Here's how the part is built. I have some questions about the finished solid (model axes, mm). Face numbers are marked on the shaded views. A direction names the side the tool comes from. Round coordinates to 2 decimals unless told otherwise and drop trailing zeros. Order: outer loops, then holes, each group sorted by start corner. A loop starts at its lowest first (then second) coordinate and runs counter-clockwise, first axis right, second up.
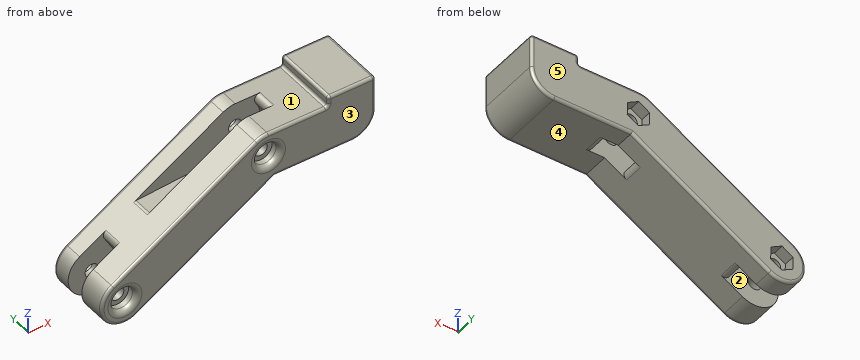
```python
from build123d import *

# Parameters (mm, degrees)
SKETCH1_R               = 1.2
BOSS_EXTRUDE1_DEPTH     = 12
CUT_EXTRUDE1_DEPTH      = 2.5
CUT_EXTRUDE1_DEPTH_BACK = 1
CUT_EXTRUDE2_DEPTH      = 2
SKETCH5_R               = 2.05
CUT_EXTRUDE3_DEPTH      = 2
FILLET1_R               = 1
FILLET2_R               = 0.5


with BuildPart() as part:
    # Sketch1 → Boss-Extrude1 (new body)
    with BuildSketch(Plane(origin=(0, 0, 0), x_dir=(1, 0, 0), z_dir=(0, 1, 0))):
        with BuildLine():
            Line((1.323018794, 17.222814504), (26.105840038, 2.488576956))
            Line((26.105840038, 2.488576956), (39.937870576, 2.488576956))
            ThreePointArc((39.937870576, 2.488576956), (42.943074396, 1.243780776), (44.187870576, -1.761423044))
            Line((44.187870576, -1.761423044), (44.187870576, -7.85))
            Line((44.187870576, -7.85), (35.687870576, -7.85))
            Line((35.687870576, -7.85), (35.687870576, -6.011423044))
            Line((35.687870576, -6.011423044), (24.937870576, -6.011423044))
            ThreePointArc((24.937870576, -6.011423044), (23.811655258, -5.859488326), (22.76596286, -5.414547306))
            Line((22.76596286, -5.414547306), (-3.020796638, 9.91656598))
            ThreePointArc((-3.020796638, 9.91656598), (-4.502013184, 15.741597958), (1.323018794, 17.222814504))
        make_face()
        with Locations(Location((-0.848888922, 13.569690242, 0), (0, 0, 270))):
            Circle(SKETCH1_R, mode=Mode.SUBTRACT)
        with Locations(Location((24.937870576, -1.761423044, 0), (0, 0, 270))):
            Circle(SKETCH1_R, mode=Mode.SUBTRACT)
    extrude(amount=BOSS_EXTRUDE1_DEPTH)

    # Sketch3 → Cut-Extrude1 (cut, two sides: drawn at the far end of the back side and taken through both)
    with BuildSketch(Plane(origin=(0, 6, 0), x_dir=(1, 0, 0), z_dir=(0, 1, 0)).offset(-CUT_EXTRUDE1_DEPTH_BACK)):
        with BuildLine():
            Line((-22.892544244, 0.947199994), (-3.741433166, 17.016890236))
            ThreePointArc((-3.741433166, 17.016890236), (2.065644543, 16.998318931), (3.019125003, 11.270023249))
            Line((3.019125003, 11.270023249), (-1.084785494, 4.367292117))
            ThreePointArc((-1.084785494, 4.367292117), (-0.38864398, 4.483185905), (0.317056148, 4.488816704))
            Line((0.317056148, 4.488816704), (25.254926724, 2.72739366))
            ThreePointArc((25.254926724, 2.72739366), (28.925298394, 0.324342858), (28.805884501, -4.061090037))
            Line((28.805884501, -4.061090037), (16.029956762, -25.550056285))
            ThreePointArc((16.029956762, -25.550056285), (9.862275844, -27.118403217), (8.293928913, -20.950722299))
            Line((8.293928913, -20.950722299), (17.339631919, -5.735951945))
            Line((17.339631919, -5.735951945), (-0.317056148, -4.488816704))
            ThreePointArc((-0.317056148, -4.488816704), (-2.876129239, -3.460907482), (-4.354991754, -1.1331579))
            Line((-4.354991754, -1.1331579), (-9.756802736, -10.218942999))
            ThreePointArc((-9.756802736, -10.218942999), (-15.508332614, -12.006129032), (-17.885892009, -6.472473713))
            ThreePointArc((-17.885892009, -6.472473713), (-23.730198417, -5.017065706), (-22.892544244, 0.947199994))
        make_face()
    extrude(amount=CUT_EXTRUDE1_DEPTH + CUT_EXTRUDE1_DEPTH_BACK, mode=Mode.SUBTRACT)

    # Sketch4 → Cut-Extrude2 (cut)
    with BuildSketch(Plane(origin=(0, 12, 0), x_dir=(1, 0, 0), z_dir=(0, 1, 0))):
        Polygon((22.952804904, -0.581233393), (22.923263521, -2.890445518), (24.908329193, -4.07063517), (26.922936248, -2.941612695), (26.952477631, -0.63240057), (24.967411959, 0.547789081), align=None)
        Polygon((1.13617675, 12.389500591), (1.165718133, 14.698712717), (-0.819347539, 15.878902368), (-2.833954594, 14.749879893), (-2.863495977, 12.440667768), (-0.878430305, 11.260478117), align=None)
    extrude(amount=-CUT_EXTRUDE2_DEPTH, mode=Mode.SUBTRACT)

    # Sketch5 → Cut-Extrude3 (cut)
    with BuildSketch(Plane.XZ):
        with Locations(Location((-0.848888922, -13.569690242, 0), (0, 0, 270))):
            Circle(SKETCH5_R)
        with Locations(Location((24.937870576, 1.761423044, 0), (0, 0, 270))):
            Circle(SKETCH5_R)
    extrude(amount=-CUT_EXTRUDE3_DEPTH, mode=Mode.SUBTRACT)

    # Fillet1
    # the kernel refuses this fillet: 1 mm, written as the material it takes off along each edge
    with BuildSketch(Plane(origin=(26.416890522, 8.5, -2.488576956), x_dir=(1, 0, 0), z_dir=(0, -1, 0)), Plane(origin=(2.594323181, 8.5, -16.466980426), x_dir=(0.8595586499303869, 0, 0.511037109542791), z_dir=(0, -1, 0))) as fillet1_piece_1:
        with BuildLine():
            CenterArc((2.958039892, 1), FILLET1_R, 143.77845338, 126.22154662)
            ThreePointArc((2.151301739, 1.590909091), (1.196627809, 0.631863865), (0, 0))
            Line((0, 0), (2.958039892, 0))
        make_face()
    extrude(amount=3.5, mode=Mode.SUBTRACT)
    with BuildSketch(Plane(origin=(27.64634461, 5, 6.011423044), x_dir=(1, 0, 0), z_dir=(0, 1, 0))) as fillet1_piece_2:
        with BuildLine():
            CenterArc((FILLET1_R * 1.75792205647, FILLET1_R), FILLET1_R, 149.267064192, 120.732935808)
            Line((FILLET1_R * 0.89836340654, FILLET1_R * 1.51103710954), (0, 0))
            Line((0, 0), (FILLET1_R * 1.75792205647, 0))
        make_face()
    extrude(amount=3.5, mode=Mode.SUBTRACT)
    with BuildSketch(Plane(origin=(6.889434617, 8.5, -4.024593471), x_dir=(-0.8595586499303914, 0, -0.5110371095427833), z_dir=(0, -1, 0))) as fillet1_piece_3:
        with BuildLine():
            CenterArc((FILLET1_R * 0.237244349344, FILLET1_R), FILLET1_R, 243.307295898, 26.692704102)
            Line((-FILLET1_R * 0.211960885996, FILLET1_R * 0.10657140378), (0, 0))
            Line((0, 0), (FILLET1_R * 0.237244349344, 0))
        make_face()
    extrude(amount=3.5, mode=Mode.SUBTRACT)
    with BuildSketch(Plane(origin=(0.847217287, 5, -7.616898987), x_dir=(0.8595586499303871, 0, 0.5110371095427908), z_dir=(0, 1, 0))) as fillet1_piece_4:
        with BuildLine():
            CenterArc((FILLET1_R, FILLET1_R), FILLET1_R, 180, 90)
            Line((0, FILLET1_R), (0, 0))
            Line((0, 0), (FILLET1_R, 0))
        make_face()
    extrude(amount=3.5, mode=Mode.SUBTRACT)
    with BuildSketch(Plane(origin=(25.838473904, 8.5, -2.647535296), x_dir=(-0.8595586499303872, 0, -0.5110371095427904), z_dir=(0, -1, 0))) as fillet1_piece_5:
        with BuildLine():
            CenterArc((4.300870532, -1), FILLET1_R, 90, 153.307295898)
            Line((3.851665297, -1.893428596), (3.806744773, -1.982771456))
            ThreePointArc((3.806744773, -1.982771456), (0.49748309, -0.318914177), (-0.03286711, -0.094444444))
            Line((-0.03286711, -0.094444444), (0, 0.1))
            Line((0, 0.1), (4.300870532, 0.1))
            Line((4.300870532, 0.1), (4.300870532, 0))
        make_face()
    extrude(amount=3.5, mode=Mode.SUBTRACT)
    with BuildSketch(Plane(origin=(24.937870576, 0, 1.761423044), x_dir=(0, 0, -1), z_dir=(-1, 0, 0))) as fillet1_piece_6:
        with BuildLine():
            CenterArc((2.05 + FILLET1_R, -FILLET1_R), FILLET1_R, 90, 90)
            Line((2.05, -FILLET1_R), (2.05, 0))
            Line((2.05, 0), (2.05 + FILLET1_R, 0))
        make_face()
    revolve(axis=Axis((24.937870576, 0, 1.761423044), (0, -1, 0)), mode=Mode.SUBTRACT)
    with BuildSketch(Plane(origin=(-0.848888922, 0, -13.569690242), x_dir=(0, 0, -1), z_dir=(-1, 0, 0))) as fillet1_piece_7:
        with BuildLine():
            CenterArc((2.05 + FILLET1_R, -FILLET1_R), FILLET1_R, 90, 90)
            Line((2.05, -FILLET1_R), (2.05, 0))
            Line((2.05, 0), (2.05 + FILLET1_R, 0))
        make_face()
    revolve(axis=Axis((-0.848888922, 0, -13.569690242), (0, -1, 0)), mode=Mode.SUBTRACT)

    # Fillet2
    fillet2_edges = [part.edges().sort_by_distance(p)[0] for p in [
        (-4.502013184, 0, -15.741597958),
        (13.714429416, 0, -9.85569573),
        (33.021855307, 0, -2.488576956),
        (42.943074396, 0, -1.243780776),
        (44.187870576, 0, 4.805711522),
        (39.937870576, 0, 7.85),
        (35.687870576, 0, 6.930711522),
        (30.312870576, 0, 6.011423044),
        (9.872583111, 12, -2.251009337),
        (23.811655258, 0, 5.859488326),
        (9.872583111, 0, -2.251009337),
        (23.811655258, 12, 5.859488326),
        (44.187870576, 6, 7.85),
        (35.687870576, 6, 7.85),
        (35.687870576, 6, 6.011423044),
        (30.312870576, 12, 6.011423044),
        (35.687870576, 12, 6.930711522),
        (39.937870576, 12, 7.85),
        (44.187870576, 12, 4.805711522),
        (42.943074396, 12, -1.243780776),
        (33.021855307, 12, -2.488576956),
        (13.714429416, 12, -9.85569573),
        (-4.502013184, 12, -15.741597958),
    ]]
    fillet(fillet2_edges, radius=FILLET2_R)


solid = part.part
```
1. If we section it at B-B, the plane y = 3: Write out the boundary of the cut face in (x, z), and give its area (3 significant figures).
Evaluation:
outline: (-3.02, -9.92) arc R4.25 ccw to (1.32, -17.22) - (26.11, -2.49) - (39.94, -2.49) arc R4.25 ccw to (44.19, 1.76) - (44.19, 7.35) arc R0.5 ccw to (43.69, 7.85) - (36.19, 7.85) arc R0.5 ccw to (35.69, 7.35) - (35.69, 6.51) arc R0.5 cw to (35.19, 6.01) - (24.94, 6.01) arc R4.25 ccw to (22.77, 5.41) - close; hole circle Ø2.4 at (-0.85, -13.57); hole circle Ø2.4 at (24.94, 1.76)
area: 450 mm2
2. If we section it at A-A, the plane x = 37.5: Write out the boundary of the cut face in (y, z), and give its area (3 significant figures).
Evaluation:
outline: (0, -1.99) arc R0.5 ccw to (0.5, -2.49) - (11.5, -2.49) arc R0.5 ccw to (12, -1.99) - (12, 7.35) arc R0.5 ccw to (11.5, 7.85) - (0.5, 7.85) arc R0.5 ccw to (0, 7.35) - close
area: 124 mm2
3. I need wall thicknesses on probe 1 along Y at (x, z) = (1, -8.5); probe 2 along Z at (x, y) = (38, 6.5); probe 3 along X at (y, z) = (1.5, 2.5). Which ranges of each line are inside material? Lowest first, please.
Evaluation:
probe 1: y = 0 to 5, 8.5 to 12
probe 2: z = -2.49 to 7.85
probe 3: x = 17.86 to 23.03, 26.85 to 44.19
4. On a 3-axis mill with a long thin cutter (end or side, diameter ignored), from which of +Z, -Z, +X, -X, +Y, -Y can I reach the whole of each face in a straight line? I mean the marked faces 1, 2, 3, 4 and 5. Say none if no direction works.
Evaluation:
face 1: +Z, -X, +Y, -Y
face 2: -Z, -X
face 3: +Z, -Z, +X, -X, -Y
face 4: -Z, +X, +Y, -Y
face 5: +Z, -Z, +X, -X, +Y
5. I'm going to push flat-ended pins straight in: P1, Ø5.5, axis at x = -0.85, z = -13.57, coming from the -Y side; P2, Ø5, axis at x = 32.5, y = 8, coming from the +Z side; P3, Ø3.5, axis at x = 34.5, y = 3.5, coming from the -Z side. Where does each tip first touch, or does it pass through?
Evaluation:
P1: stops at y = 0.05
P2: stops at z = 6.01
P3: stops at z = -2.49
